from build123d import *

# Parameters (mm, degrees)
SKETCH_1_R      = 2.1
SKETCH_1_R_2    = 1
EXTRUDE_1_DEPTH = 4.2
SKETCH_2_R      = 3
SKETCH_2_R_2    = 2.1
EXTRUDE_3_DEPTH = 1
FILLET_1_R      = 0.3


with BuildPart() as part:
    # 草图1 → 凸台-拉伸1 (new body)
    with BuildSketch(Plane(origin=(0, 0, 0), x_dir=(1, 0, 0), z_dir=(0, 1, 0))):
        Circle(SKETCH_1_R)
        Circle(SKETCH_1_R_2, mode=Mode.SUBTRACT)
    extrude(amount=EXTRUDE_1_DEPTH)

    # 草图2 → 凸台-拉伸3 (add)
    with BuildSketch(Plane(origin=(0, 4.2, 0), x_dir=(1, 0, 0), z_dir=(0, 1, 0))):
        Circle(SKETCH_2_R)
        Circle(SKETCH_2_R_2, mode=Mode.SUBTRACT)
    extrude(amount=-EXTRUDE_3_DEPTH)

    # 圆角1
    fillet_1_edges = [part.edges().sort_by_distance(p)[0] for p in [
        (-3, 4.2, 0),
        (-1, 4.2, 0),
    ]]
    fillet(fillet_1_edges, radius=FILLET_1_R)


solid = part.part
The listing builds one solid part. Answer for the finished solid, in the listing's coordinates (mm). Round coordinates to 2 decimals unless told otherwise and drop trailing zeros. Write each loop counter-clockwise with the first axis right and the second up, starting at its lowest first coordinate (ties: lowest second). Pieces come first, ordered by that corner, then holes. Notation, with made-up numbers: M -18.5,86 L 33.5,86 A21 cw 33.5,117 Z; hole C 70,-31.5 d3. An arc over 180 degrees is marked long. Write each question's results on one line, items separated by ' | '. Start each with the question number.
Item 1: Find section C-C on y = 1.15. Write down the section's boundary in (x, z).
Item 2: Given pin 1 Ø2 at (y, z) = (2.5, -1) entering from +X; pin 2 Ø1 at (y, z) = (3.5, -2) entering from +X, each flat-ended and moving along its own axis, determine where each tip first touches the part or whether it passes through.
Item 3: Straight lines are drawn through the part: probe 1 along X at (y, z) = (2.3, 0); probe 2 along Y at (x, z) = (0, -2.5). For each, find the intervals that lie inside material, in ascending order.
Item 4: The mould has two halves that part along X. Classify faces 1 (the cylindrical face through (0, 2, 1)), 2 (the flat face through (1.3, 3.2, 2)), 3 (the cylindrical face through (2.003, 1.578, -0.631)): +X half, -X half, draft (parallel to the pull), parting line (faces both ways), or undercut.
Item 5: Find section B-B on x = 0. Write down the section's boundary in (y, z), and give its area (3 significant figures).
Item 6: Find section A-A on z = 0. Write down the section's boundary in (x, y), and give its area (3 significant figures).
Answer block:
1) outline: C 0,0 d4.2; hole C 0,0 d2
2) pin 1: stops at x = 2.99 | pin 2: stops at x = 2.6
3) probe 1: x = -2.1 to -1, 1 to 2.1 | probe 2: y = 3.2 to 4.2
4) face 1: undercut | face 2: draft | face 3: parting line
5) outline: M 0,-2.1 L 3.2,-2.1 L 3.2,-3 L 3.9,-3 A0.3 ccw 4.2,-2.7 L 4.2,-1.3 A0.3 ccw 3.9,-1 L 0,-1 Z; M 0,1 L 3.9,1 A0.3 ccw 4.2,1.3 L 4.2,2.7 A0.3 ccw 3.9,3 L 3.2,3 L 3.2,2.1 L 0,2.1 Z | area: 11.0 mm²
6) outline: M -3,3.2 L -2.1,3.2 L -2.1,0 L -1,0 L -1,3.9 A0.3 ccw -1.3,4.2 L -2.7,4.2 A0.3 ccw -3,3.9 Z; M 1,0 L 2.1,0 L 2.1,3.2 L 3,3.2 L 3,3.9 A0.3 ccw 2.7,4.2 L 1.3,4.2 A0.3 ccw 1,3.9 Z | area: 11.0 mm²
